Here's how the part is built. I have some questions about the finished solid (model axes, mm). Round coordinates to 2 decimals unless told otherwise and drop trailing zeros. Loops run counter-clockwise (first coordinate to the right, second up) from the corner with the lowest first, then second, coordinate; pieces in that order, holes last. Notation, with made-up numbers: M 40,68.25 L 65,68.25 A25 ccw 65,90.25 Z; hole C 4,-38 d4. An arc over 180 degrees is marked long. Answer as a JSON object with one key per item and string values.
from build123d import *
from OCP.BRepFilletAPI import BRepFilletAPI_MakeChamfer

# Parameters (mm, degrees)
CHAMFER1_SIZE  = 0.5
CHAMFER2_SIZE  = 0.5
CHAMFER2_SIZE2 = 0.288675135


with BuildPart() as part:
    # Sketch1 → Revolve1 (revolve)
    with BuildSketch(Plane.XY):
        Polygon((-8, -51), (-8, -589), (-5, -589), (-5, -597), (-4.8, -597), (-4.8, -598.15), (-5, -598.15), (-5, -600), (-1, -600), (-1, -597), (0, -597), (0, -3), (-1, -3), (-1, 0), (-5, 0), (-5, -15), (-6, -15), (-6, -51), align=None)
    revolve(axis=Axis((0, -3, 0), (0, -1, 0)))

    # Chamfer1
    chamfer1_edges = [part.edges().sort_by_distance(p)[0] for p in [
        (6, -15, 0),
        (8, -51, 0),
        (8, -589, 0),
        (5, -600, 0),
        (5, 0, 0),
    ]]
    chamfer(chamfer1_edges, length=CHAMFER1_SIZE)

    # Chamfer2: one chamfer whose edges measure the first distance from different faces: ONE call of the kernel's chamfer builder (chamfer() names one face for all edges)
    chamfer2_edges_1 = [part.edges().sort_by_distance(p)[0] for p in [
        (1, -600, 0),
    ]]
    chamfer2_side_1 = [part.faces().sort_by_distance(p)[0] for p in [
        (1, -598.5, 0),
    ]]
    chamfer2_edges_2 = [part.edges().sort_by_distance(p)[0] for p in [
        (1, -597, 0),
    ]]
    chamfer2_side_2 = [part.faces().sort_by_distance(p)[0] for p in [
        (0, -597, 0),
    ]]
    chamfer2_edges_3 = [part.edges().sort_by_distance(p)[0] for p in [
        (1, -3, 0),
    ]]
    chamfer2_side_3 = [part.faces().sort_by_distance(p)[0] for p in [
        (1, -1.5, 0),
    ]]
    chamfer2_edges_4 = [part.edges().sort_by_distance(p)[0] for p in [
        (1, 0, 0),
    ]]
    chamfer2_side_4 = [part.faces().sort_by_distance(p)[0] for p in [
        (4.372720779, 0, 0),
    ]]
    chamfer2 = BRepFilletAPI_MakeChamfer(part.part.solid().wrapped)
    for e in chamfer2_edges_1:
        chamfer2.Add(CHAMFER2_SIZE, CHAMFER2_SIZE2, e.wrapped, chamfer2_side_1[0].wrapped)  # the first distance lies on this face
    for e in chamfer2_edges_2:
        chamfer2.Add(CHAMFER2_SIZE, CHAMFER2_SIZE2, e.wrapped, chamfer2_side_2[0].wrapped)  # the first distance lies on this face
    for e in chamfer2_edges_3:
        chamfer2.Add(CHAMFER2_SIZE, CHAMFER2_SIZE2, e.wrapped, chamfer2_side_3[0].wrapped)  # the first distance lies on this face
    for e in chamfer2_edges_4:
        chamfer2.Add(CHAMFER2_SIZE, CHAMFER2_SIZE2, e.wrapped, chamfer2_side_4[0].wrapped)  # the first distance lies on this face
    add(Compound.cast(chamfer2.Shape()), mode=Mode.REPLACE)


solid = part.part
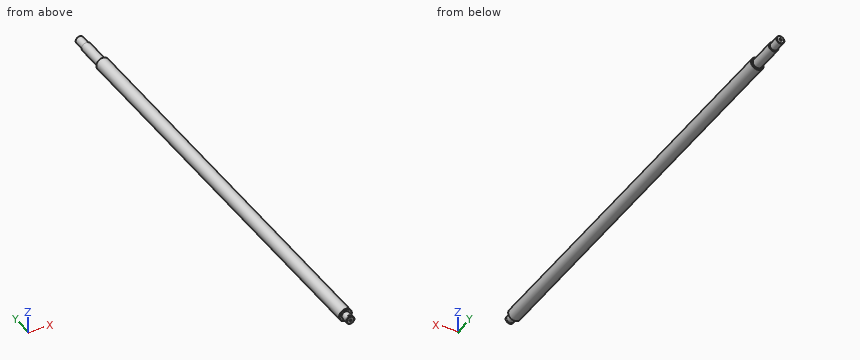
Item 1: Please list where these lines run through material, in increasing order: probe 1 along Z at (x, y) = (0, -1.5); probe 2 along Z at (x, y) = (0, -597.9). Write a range as from..to.
Resolved:
{"probe 1": "-5..-1, 1..5", "probe 2": "-4.8..-1, 1..4.8"}
Item 2: I want a section at A-A, the plane y = -465.5. Please give me the cut outline in (x, z).
Resolved:
{"outline": "C 0,0 d16"}
Item 3: I'm going to push flat-ended pins straight in: pin 1 Ø3 at (x, z) = (0.5, 2) entering from +Y; pin 2 Ø1.6 at (x, z) = (0, 0) entering from +Y; pin 3 Ø1.8 at (x, z) = (0, 0) entering from -Y; pin 4 Ø5 at (y, z) = (-305, 3.5) entering from -X. Where does each tip first touch, or does it pass through?
Resolved:
{"pin 1": "y = 0", "pin 2": "y = -2.85", "pin 3": "y = -597.23", "pin 4": "x = -7.94"}
